Autodesk Inventor part; units mm, degrees
ref_plane "YZ Plane" through (0, 0, 0) normal (1, 0, 0) x (0, 1, 0)
ref_plane "XZ Plane" through (0, 0, 0) normal (0, 1, 0) x (-1, 0, 0)
ref_plane "XY Plane" through (0, 0, 0) normal (0, 0, 1) x (1, 0, 0)
sketch "Skizze1" plane through (0, 0, 0) normal (0, 1, 0) x (-1, 0, 0)
  circle A0 centre (0, 0) radius 5
  circle A1 centre (0, 0) radius 3
  dimension "d0" = 10
  dimension "d1" = 6
extrude "Extrusion1" add sketch "Skizze1" along normal mid plane 12
fillet "Rundung1" radius 1 2 edges at (5, -6, 0) (5, 6, 0)
properties part number "BromzeFitting" material "Bronze, Guss"
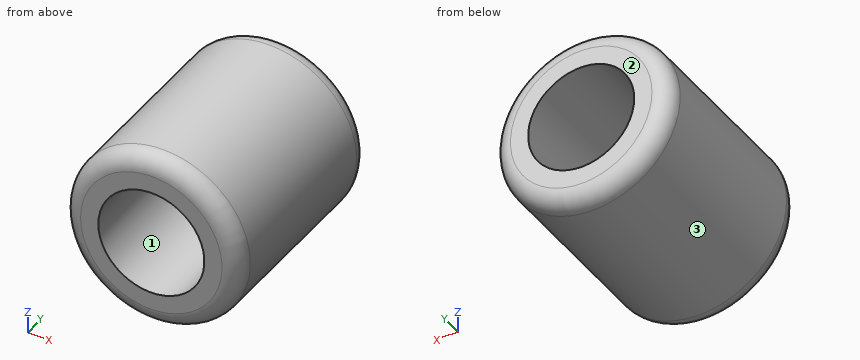
Part model, mm, in its own coordinate system. Face numbers are marked on the shaded views. Coordinates: 2 decimals unless noted, no trailing zeros. Order: outer loops, then holes, each group sorted by start corner. A loop starts at its lowest first (then second) coordinate and runs counter-clockwise, first axis right, second up. Notation, with made-up numbers: M -6.75,22.5 L 20.25,22.5 A21 cw 20.25,47.5 Z; hole C -11,28.25 d1. An arc over 180 degrees is marked long. Use a Markdown table: item, result.
(1) Pull direction X, two halves, no side cores. Call the marked faces 1, 2 and 3: released by +X, released by -X, zero draft, split by the parting line, or undercut.
A:
| item | result |
|---|---|
| face 1 | undercut |
| face 2 | zero draft |
| face 3 | split by the parting line |
(2) Probe L1, parallel to Z at x = 0, y = -0.75; L2, parallel to X at y = 4.5, z = -1.75; L3, parallel to X at y = -5.25, z = 2.5. List the from-to ranges inside material, lowest first.
A:
| item | result |
|---|---|
| L1 | z = -5 to -3, 3 to 5 |
| L2 | x = -4.68 to -2.44, 2.44 to 4.68 |
| L3 | x = -4.29 to -1.66, 1.66 to 4.29 |
(3) Cut at C-C on y = -3.5. Write the cut outline in (x, z), then the cut area to 3 significant figures.
A:
| item | result |
|---|---|
| outline | C 0,0 d10; hole C 0,0 d6 |
| area | 50.3 mm^2 |
(4) Flat gauge pins, fed straight in: pin 1 (3 mm diameter, centred on x = -2, y = 1.5, fed in from -Z); pin 2 (5 mm diameter, centred on x = 0, z = 0, fed in from -Y). Where does each tip first touch, or does it go through?
A:
| item | result |
|---|---|
| pin 1 | stops at z = -4.97 |
| pin 2 | passes through |
(5) Cut at B-B on z = 0. Write the cut outline in (x, y).
A:
| item | result |
|---|---|
| outline | M -5,-5 A1 ccw -4,-6 L -3,-6 L -3,6 L -4,6 A1 ccw -5,5 Z; M 3,-6 L 4,-6 A1 ccw 5,-5 L 5,5 A1 ccw 4,6 L 3,6 Z |
(6) Cut at A-A on x = 0. Write the cut outline in (y, z), then the cut area to 3 significant figures.
A:
| item | result |
|---|---|
| outline | M -6,-4 A1 ccw -5,-5 L 5,-5 A1 ccw 6,-4 L 6,-3 L -6,-3 Z; M -6,3 L 6,3 L 6,4 A1 ccw 5,5 L -5,5 A1 ccw -6,4 Z |
| area | 47.1 mm^2 |
